```python
from build123d import *

# Parameters (mm, degrees)
SM_BASE_FLANGE_1_DEPTH    = 100
CUT_EXTRUDE_1_DEPTH       = 1.5
SKETCH_7_R                = 2
CUT_EXTRUDE_2_DEPTH       = 1.5
CUT_EXTRUDE_START         = -10
CUT_EXTRUDE_3_OUTLINE_W   = 100
CUT_EXTRUDE_3_OUTLINE_H   = 4
CUT_EXTRUDE_3_DEPTH       = 8.5
CUT_EXTRUDE_START_2       = -1.5
CUT_EXTRUDE_3_2_DEPTH     = 1.5
CUT_EXTRUDE_3_3_OUTLINE_R = 2
CUT_EXTRUDE_3_3_DEPTH     = 1.5


# Read off the part's stored shape, not the designer's step: Вырез-Вытянуть3
# Sheet-metal steps are written as plain solids
with BuildPart() as part:
    # Sketch 1 → Базовая кромка1 (new body)
    with BuildSketch(Plane(origin=(0, 0, 0), x_dir=(0, 0, -1), z_dir=(1, 0, 0))):
        with BuildLine():
            Line((10, 0), (3, 0))
            ThreePointArc((3, 0), (0.878679656, 0.878679656), (0, 3))
            Line((0, 3), (0, 15))
            Line((0, 15), (1.5, 15))
            Line((1.5, 15), (1.5, 3))
            ThreePointArc((1.5, 3), (1.939339828, 1.939339828), (3, 1.5))
            Line((3, 1.5), (10, 1.5))
            Line((10, 1.5), (10, 0))
        make_face()
    extrude(amount=SM_BASE_FLANGE_1_DEPTH)

    # Эскиз6 → Вырез-Вытянуть1 (cut)
    with BuildSketch(Plane.XY):
        with BuildLine():
            Line((0, 11.792498505), (0, 18.792498505))
            Line((0, 18.792498505), (100, 18.792498505))
            Line((100, 18.792498505), (100, 11.792498505))
            ThreePointArc((100, 11.792498505), (94.444444444, 15), (88.888888889, 11.792498505))
            ThreePointArc((88.888888889, 11.792498505), (83.333333333, 8.584997009), (77.777777778, 11.792498505))
            ThreePointArc((77.777777778, 11.792498505), (72.222222222, 15), (66.666666667, 11.792498505))
            ThreePointArc((66.666666667, 11.792498505), (61.111111111, 8.584997009), (55.555555556, 11.792498505))
            ThreePointArc((55.555555556, 11.792498505), (50, 15), (44.444444444, 11.792498505))
            ThreePointArc((44.444444444, 11.792498505), (38.888888889, 8.584997009), (33.333333333, 11.792498505))
            ThreePointArc((33.333333333, 11.792498505), (27.777777778, 15), (22.222222222, 11.792498505))
            ThreePointArc((22.222222222, 11.792498505), (16.666666667, 8.584997009), (11.111111111, 11.792498505))
            ThreePointArc((11.111111111, 11.792498505), (5.555555556, 15), (0, 11.792498505))
        make_face()
    extrude(amount=-CUT_EXTRUDE_1_DEPTH, mode=Mode.SUBTRACT)

    # Эскиз7 → Вырез-Вытянуть2 (cut)
    with BuildSketch(Plane(origin=(0, 1.5, 0), x_dir=(1, 0, 0), z_dir=(0, 1, 0))):
        with Locations(Location((50, 6.5, 0), (0, 0, 270))):
            Circle(SKETCH_7_R)
        with Locations(Location((95, 6.5, 0), (0, 0, 270))):
            Circle(SKETCH_7_R)
        with Locations(Location((5, 6.5, 0), (0, 0, 270))):
            Circle(SKETCH_7_R)
    extrude(amount=-CUT_EXTRUDE_2_DEPTH, mode=Mode.SUBTRACT)

    # Вырез-Вытянуть3 outline → Вырез-Вытянуть3 (cut)
    with BuildSketch(Plane.XY.offset(CUT_EXTRUDE_START)):
        with Locations((50, 2)):
            Rectangle(CUT_EXTRUDE_3_OUTLINE_W, CUT_EXTRUDE_3_OUTLINE_H)
    extrude(amount=CUT_EXTRUDE_3_DEPTH, mode=Mode.SUBTRACT)

    # Cut-Extrude 3 2 outline → Cut-Extrude 3 2 (cut)
    with BuildSketch(Plane.XY.offset(CUT_EXTRUDE_START_2)):
        with BuildLine():
            ThreePointArc((0, 0.232854132), (1, 1.232854132), (0, 2.232854132))
            Line((0, 2.232854132), (0, 0.232854132))
        make_face()
        with BuildLine():
            Line((100, 0.232854132), (100, 2.232854132))
            ThreePointArc((100, 2.232854132), (99, 1.232854132), (100, 0.232854132))
        make_face()
    extrude(amount=CUT_EXTRUDE_3_2_DEPTH, mode=Mode.SUBTRACT)

    # Cut-Extrude 3 3 outline → Cut-Extrude 3 3 (add)
    with BuildSketch(Plane.XY.offset(CUT_EXTRUDE_START_2)):
        with BuildLine():
            Line((0, 0.232854132), (0, -7.534291735))
            Line((0, -7.534291735), (100, -7.534291735))
            Line((100, -7.534291735), (100, 0.232854132))
            ThreePointArc((100, 0.232854132), (99, 1.232854132), (100, 2.232854132))
            Line((100, 2.232854132), (100, 4))
            Line((100, 4), (0, 4))
            Line((0, 4), (0, 2.232854132))
            ThreePointArc((0, 2.232854132), (1, 1.232854132), (0, 0.232854132))
        make_face()
        with Locations((95, -4.034291735)):
            Circle(CUT_EXTRUDE_3_3_OUTLINE_R, mode=Mode.SUBTRACT)
        with Locations((5, -4.034291735)):
            Circle(CUT_EXTRUDE_3_3_OUTLINE_R, mode=Mode.SUBTRACT)
        with Locations((50, -4.034291735)):
            Circle(CUT_EXTRUDE_3_3_OUTLINE_R, mode=Mode.SUBTRACT)
    extrude(amount=CUT_EXTRUDE_3_3_DEPTH)


solid = part.part
```
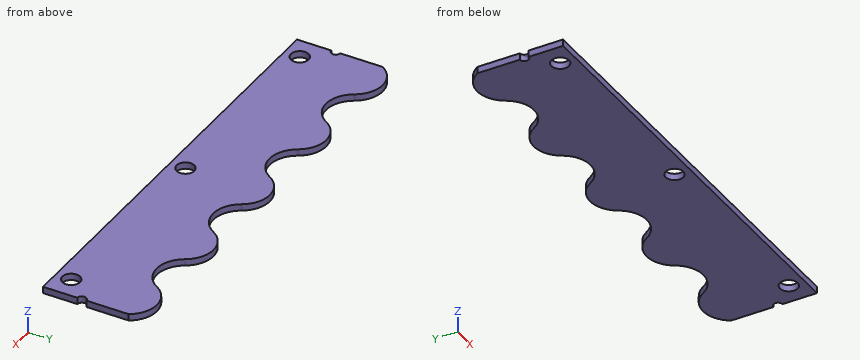
Geometry check sheet. Reference: the model listing, model coordinates, mm. Give positions to 0.01 mm unless a question says otherwise; leave off trailing zeros. Write each loop counter-clockwise with the first axis right and the second up, starting at its lowest first coordinate (ties: lowest second). Pieces come first, ordered by that corner, then holes. Notation, with made-up numbers: (12.5, 18.25) - (65.5, 18.25) arc R13 cw to (65.5, 28.25) - close; hole circle Ø1 at (-12.75, 19). An arc over 180 degrees is marked (long way). Use a Markdown table: item, result.
Q1. Thickness scan on L1, parallel to X at y = -5.5, z = -0.6; L2, parallel to Y at x = 50, z = -1; L3, parallel to X at y = 13, z = -1.15. Record the ranges inside material, lowest first. Write a range as [from, to].
Computed:
| item | result |
|---|---|
| L1 | x = [0, 3.64], [6.36, 48.64], [51.36, 93.64], [96.36, 100] |
| L2 | y = [-7.53, -6.03], [-2.03, 15] |
| L3 | x = [0.9, 10.21], [23.12, 32.43], [45.35, 54.65], [67.57, 76.88], [89.79, 99.1] |
Q2. Section check A-A, the plane x = 95. Enter the section's corners in (y, z), then the cut area to 3 significant figures.
Computed:
| item | result |
|---|---|
| outline | (-7.53, -1.5) - (-6.03, -1.5) - (-6.03, 0) - (-7.53, 0) - close; (-2.03, -1.5) - (14.98, -1.5) - (14.98, 0) - (-2.03, 0) - close |
| area | 27.8 mm² |
Q3. Section check D-D, the plane x = 65. Enter the section's corners in (y, z), then the cut area to 3 significant figures.
Computed:
| item | result |
|---|---|
| outline | (-7.53, -1.5) - (9.9, -1.5) - (9.9, 0) - (-7.53, 0) - close |
| area | 26.1 mm² |
Q4. Go/stop test with a flat-tipped pin: P1, Ø2.5, axis at x = 5, y = -4.03, coming from the +Z side. Record where the tip stops, or that it passes through.
Computed:
| item | result |
|---|---|
| P1 | passes through |
Q5. Section check C-C, the plane x = 32. Enter the section's corners in (y, z), then the cut area to 3 significant figures.
Computed:
| item | result |
|---|---|
| outline | (-7.53, -1.5) - (13.41, -1.5) - (13.41, 0) - (-7.53, 0) - close |
| area | 31.4 mm² |
Q6. Section check B-B, the plane z = -0.85. Enter the section's corners in (x, y) (1 decimal).
Computed:
| item | result |
|---|---|
| outline | (0, -7.5) - (100, -7.5) - (100, 0.2) arc R1 cw to (100, 2.2) - (100, 11.8) arc R6.4 ccw to (88.9, 11.8) arc R6.4 cw to (77.8, 11.8) arc R6.4 ccw to (66.7, 11.8) arc R6.4 cw to (55.6, 11.8) arc R6.4 ccw to (44.4, 11.8) arc R6.4 cw to (33.3, 11.8) arc R6.4 ccw to (22.2, 11.8) arc R6.4 cw to (11.1, 11.8) arc R6.4 ccw to (0, 11.8) - (0, 2.2) arc R1 cw to (0, 0.2) - close; hole circle Ø4 at (5, -4); hole circle Ø4 at (50, -4); hole circle Ø4 at (95, -4) |
